Part model, mm, in its own coordinate system. A direction names the side the tool comes from. Round coordinates to 2 decimals unless told otherwise and drop trailing zeros. Write each loop counter-clockwise with the first axis right and the second up, starting at its lowest first coordinate (ties: lowest second). Pieces come first, ordered by that corner, then holes.
Autodesk Inventor part; units mm, degrees
ref_plane "YZ Plane" through (0, 0, 0) normal (1, 0, 0) x (0, 1, 0)
ref_plane "XZ Plane" through (0, 0, 0) normal (0, 1, 0) x (-1, 0, 0)
ref_plane "XY Plane" through (0, 0, 0) normal (0, 0, 1) x (1, 0, 0)
sketch "Szkic1" plane through (0, 0, 0) normal (0, 1, 0) x (-1, 0, 0)
  line L0 (0, 0) -> (12, 0)
  line L1 (12, 0) -> (12, 22)
  line L2 (12, 22) -> (0, 22)
  line L3 (0, 22) -> (0, 0)
  dimension "d0" = 12
  dimension "d1" = 22
extrude "Wyciągnięcie proste1" add sketch "Szkic1" along normal blind 22
sketch "Szkic2" plane through (-12, 0, 22) normal (0, 0, 1) x (1, 0, 0)
  line L0 (0, 0) -> (0, 22)
  line L1 (12, 0) -> (12, 22)
  line L2 (0, 18) -> (12, 18)
  line L3 (12, 18) -> (12, 16)
  line L4 (12, 16) -> (0, 16)
  line L5 (0, 16) -> (0, 18)
  line L6 (0, 22) -> (12, 22)
  dimension "d4" = 2
  dimension "d5" = 4
extrude "Wyciągnięcie proste2" add sketch "Szkic2" along normal blind 5 contours L0 L2 L1 L4
sketch "Szkic3" plane through (0, 0, 0) normal (0, 0, -1) x (-1, 0, 0)
  line L0 (0, 16) -> (0, 18)
  line L1 (12, 16) -> (0, 16)
  line L2 (0, 18) -> (12, 18)
  line L3 (12, 18) -> (12, 16)
  line L4 (12, 16) -> (0, 16)
  line L5 (0, 16) -> (0, 18)
  point P0 (0, 0)
extrude "Wyciągnięcie proste3" add sketch "Szkic3" along normal blind 5
sketch "Szkic4" plane through (-12, 18, 0) normal (0, 1, 0) x (1, 0, 0)
  line L0 (0, 5) -> (12, 5)
  point P0 (12, 0)
  point P1 (6, 2.5)
  point P2 (6, -24.839)
  dimension "d10" = 2.5
hole "Otwór1" at (-6, 18, -2.5) direction (0, -1, 0) diameter 2 end through all
sketch "Szkic5" plane through (-12, 18, 22) normal (0, 1, 0) x (1, 0, 0)
  line L0 (12, -5) -> (0, -5)
  point P0 (12, 22)
  point P1 (6, -2.5)
  dimension "d18" = 2.5
hole "Otwór2" at (-6, 18, 24.5) direction (0, -1, 0) diameter 2 end through all
sketch "Szkic6" plane through (0, 22, 0) normal (0, 1, 0) x (1, 0, 0)
  line L0 (-12, -22) -> (0, -22)
  arc A0 (-8.3077, -10.4615) -> (-3.6923, -10.4615) centre (-6, -16) ccw
  line L1 (0, 0) -> (-12, 0)
  arc A1 (-3.6923, -10.4615) -> (-8.3077, -10.4615) centre (-6, -9.5) ccw
  dimension "d26" = 6
  dimension "d27" = 9.5
  dimension "d28" = 5
extrude "Wyciągnięcie proste4" add sketch "Szkic6" along normal blind 4
sketch "Szkic7" plane through (0, 26, 0) normal (0, 1, 0) x (1, 0, 0)
  circle A0 centre (-6, -16) radius 2.5
  arc A1 (-8.3077, -10.4615) -> (-3.6923, -10.4615) centre (-6, -16) ccw
  point P0 (0, 0)
  dimension "d31" = 5
extrude "Wyciągnięcie proste5" add sketch "Szkic7" along normal blind 3
sketch "Szkic8" plane through (-12, 0, 22) normal (0, 0, 1) x (1, 0, 0)
  line L0 (4.5, 4) -> (7.5, 4)
  line L1 (8, 4.5) -> (8, 4.5)
  line L2 (7.5, 5) -> (4.5, 5)
  line L3 (4, 4.5) -> (4, 4.5)
  line L4 (0, 0) -> (12, 0)
  line L5 (12, 0) -> (12, 16)
  arc A0 (4.5, 5) -> (4, 4.5) centre (4.5, 4.5) ccw
  arc A1 (4, 4.5) -> (4.5, 4) centre (4.5, 4.5) ccw
  arc A2 (8, 4.5) -> (7.5, 5) centre (7.5, 4.5) ccw
  arc A3 (7.5, 4) -> (8, 4.5) centre (7.5, 4.5) ccw
  point P0 (8, 5)
  point P1 (8, 4)
  point P2 (4, 5)
  dimension "d34" = 4
  dimension "d35" = 1
  dimension "d36" = 4
  dimension "d37" = 4
  dimension "d38" = 0.5
extrude "Wyciągnięcie proste6" add sketch "Szkic8" along normal blind 5
properties part number "towerpro"
Q1. Cut at B-B on y = 4.5. Write the cut outline in (x, z).
Values follow:
outline: (-12, 0) - (0, 0) - (0, 22) - (-4, 22) - (-4, 27) - (-8, 27) - (-8, 22) - (-12, 22) - close
Q2. Cut at C-C on x = -1.25. Write the cut outline in (y, z), plus the area to 3 significant figures.
Values follow:
outline: (0, 0) - (16, 0) - (16, -5) - (18, -5) - (18, 0) - (22, 0) - (22, 12.33) - (26, 12.33) - (26, 19.67) - (22, 19.67) - (22, 22) - (18, 22) - (18, 27) - (16, 27) - (16, 22) - (0, 22) - close
area: 533 mm2
Q3. Which spindle directions (+Z, -Z, +X, -X, +Y, -Y) get a long thin tool onto all of the face, cutting with end or side? Do faces 1 (the cylindrical face through (-4, 4.5, 24.5)), 2 (the cylindrical face through (-3.69, 27.48, 15.04)), 3 (the flat face through (-6, 5, 24)). Say none if no direction does.
Values follow:
face 1: +Z, +X
face 2: +Y
face 3: +Z, +X, -X
Q4. Cut at D-D on z = 4. Write the cut outline in (x, y), plus the area to 3 significant figures.
Values follow:
outline: (-12, 0) - (0, 0) - (0, 22) - (-12, 22) - close
area: 264 mm2
Q5. Mould opens along Z. For faces 4 (the flat face through (-11, 22, 21)), 5 (the cylindrical face through (-6, 24, 7)), 6 (the flat face through (-6, 17, -5)), 7 (the cylindrical face through (-6.99, 16.99, 24.37)) say: +Z half, -Z half, draft (parallel to the pull), parting line (faces both ways), or undercut.
Values follow:
face 4: draft
face 5: undercut
face 6: -Z half
face 7: undercut
Q6. Wall check: L1, parallel to Z at x = -6, y = 16.9; L2, parallel to X at y = 17.65, z = 24.5; L3, parallel to Y at x = -9.25, z = 24. Give the ranges that are in metal, low to high.
Values follow:
L1: z = -5 to -3.5, -1.5 to 23.5, 25.5 to 27
L2: x = -12 to -7, -5 to 0
L3: y = 16 to 18
Q7. Cut at A-A on z = 9.5. Write the cut outline in (x, y).
Values follow:
outline: (-12, 0) - (0, 0) - (0, 22) - (-3.5, 22) - (-3.5, 26) - (-8.5, 26) - (-8.5, 22) - (-12, 22) - close
Q8. Drop flat-ended pins along their axis: pin 1 (4 mm diameter, centred on x = -8, z = -2.5, fed in from +Y); pin 2 (3 mm diameter, centred on x = -5, y = 20, fed in from -Z); pin 3 (1.5 mm diameter, centred on x = -5.5, z = 25.5, fed in from -Y). Give the stop position or say it passes through.
Values follow:
pin 1: stops at y = 18
pin 2: stops at z = 0
pin 3: stops at y = 4
